Verification items for this drawing (mm, ordinates from the low corner). A direction names the side the tool comes from. Round coordinates to 2 decimals unless told otherwise and drop trailing zeros. Write each loop counter-clockwise with the first axis right and the second up, starting at its lowest first coordinate (ties: lowest second). Pieces come first, ordered by that corner, then holes.
Item 1: Scan lines: probe 1 along Z at (x, y) = (45, 5.5); probe 2 along X at (y, z) = (5.5, 45); probe 3 along Z at (x, y) = (5, 5). Record each from-to range of solid material in increasing order.
Item 2: Access from +Z, -Z, +X, -X, +Y, -Y to the whole of each face (thin tool, end or side, straight path). Record for the marked faces 1, 2 and 3.
Item 3: Depth check by flat-ended pin: P1, Ø2.5, axis at x = 6.25, y = 35, coming from the -Z side; P2, Ø4, axis at x = 26, z = 17.5, coming from the +Y side; P3, Ø24.5, axis at x = 16, y = 35, coming from the +Z side. Enter the tip coordinate at first touch or a pass-through.
Item 4: Cross-section at C-C (y = 35). Enter the section's corners in (x, z), then the cut area to 3 significant figures.
Item 5: Cross-section at A-A (x = 55.5). Enter the section's corners in (y, z), then the cut area to 3 significant figures.
Item 6: Cross-section at B-B (z = 45). Enter the section's corners in (x, y).
Item 7: Cross-section at D-D (x = 75). Enter the section's corners in (y, z).
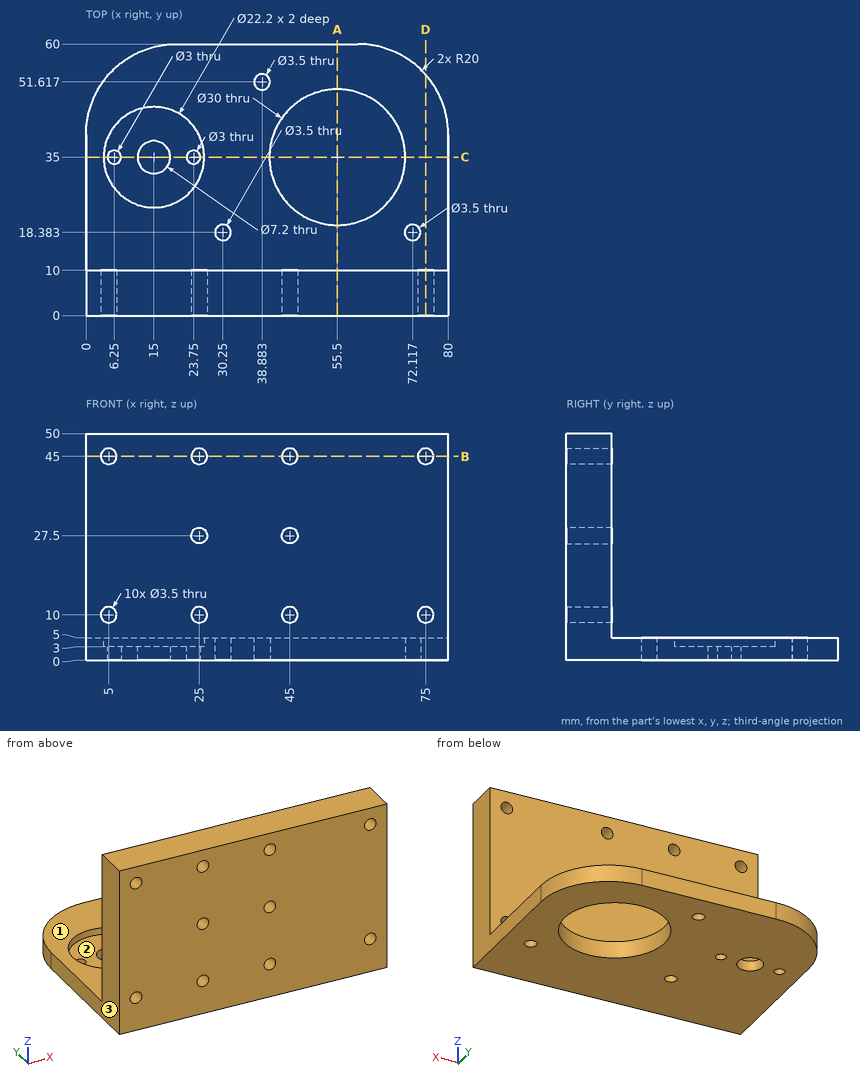
Resolved:
1. probe 1: z = 0 to 8.25, 11.75 to 25.75, 29.25 to 43.25, 46.75 to 50
1. probe 2: x = 0 to 3.25, 6.75 to 23.25, 26.75 to 43.25, 46.75 to 73.25, 76.75 to 80
1. probe 3: z = 0 to 8.25, 11.75 to 43.25, 46.75 to 50
2. face 1: +Z, +X, -X, +Y
2. face 2: +Z
2. face 3: +Z, -Z, -X, +Y, -Y
3. P1: passes through
3. P2: stops at y = 10
3. P3: stops at z = 5
4. outline: (0, 0) - (4.75, 0) - (4.75, 3) - (3.9, 3) - (3.9, 5) - (0, 5) - close; (7.75, 0) - (11.4, 0) - (11.4, 3) - (7.75, 3) - close; (18.6, 0) - (22.25, 0) - (22.25, 3) - (18.6, 3) - close; (25.25, 0) - (40.5, 0) - (40.5, 5) - (26.1, 5) - (26.1, 3) - (25.25, 3) - close; (70.5, 0) - (80, 0) - (80, 5) - (70.5, 5) - close
4. area: 166 mm2
5. outline: (0, 0) - (20, 0) - (20, 5) - (10, 5) - (10, 50) - (0, 50) - close; (50, 0) - (60, 0) - (60, 5) - (50, 5) - close
5. area: 600 mm2
6. outline: (0, 0) - (3.25, 0) - (3.25, 10) - (0, 10) - close; (6.75, 0) - (23.25, 0) - (23.25, 10) - (6.75, 10) - close; (26.75, 0) - (43.25, 0) - (43.25, 10) - (26.75, 10) - close; (46.75, 0) - (73.25, 0) - (73.25, 10) - (46.75, 10) - close; (76.75, 0) - (80, 0) - (80, 10) - (76.75, 10) - close
7. outline: (0, 0) - (53.23, 0) - (53.23, 5) - (10, 5) - (10, 8.25) - (0, 8.25) - close; (0, 11.75) - (10, 11.75) - (10, 43.25) - (0, 43.25) - close; (0, 46.75) - (10, 46.75) - (10, 50) - (0, 50) - close
